from build123d import *

# Parameters (mm, degrees)
CBORE_FOR_M3_SHCS1_D           = 3.6
CBORE_FOR_M3_SHCS1_DEPTH       = 6.500114
CBORE_FOR_M3_SHCS1_CBORE_D     = 6.5
CBORE_FOR_M3_SHCS1_CBORE_DEPTH = 3
CBORE_FOR_M3_SHCS1_TIP         = 1.081549114
CUT_EXTRUDE1_DEPTH             = 91.160967098
CUT_EXTRUDE2_DEPTH             = 93.865494063


with BuildPart() as part:
    # Sketch1 → Revolve1 (revolve)
    with BuildSketch(Plane.XY, mode=Mode.PRIVATE) as revolve1_sk:
        Polygon((0, 83.999999926), (28, 83.999999926), (28, 78.999999926), (15, 78.999999926), (15, 79.999999926), (4.5, 79.999999926), (4.5, 15), (2.5, 15), (2.5, 0), (0, 0), align=None)
    revolve(revolve1_sk.sketch.rotate(Axis((0, 0, 0), (0, 1, 0)), 90), axis=Axis((0, 0, 0), (0, 1, 0)))

    # CBORE for M3 SHCS1
    with Locations(Plane(origin=(0, 83.999999926, 0), x_dir=(1, 0, 0), z_dir=(0, 1, 0))):
        with Locations((3, 23), (-3, 23), (-3, -23), (3, -23)):
            CounterBoreHole(CBORE_FOR_M3_SHCS1_D / 2, CBORE_FOR_M3_SHCS1_CBORE_D / 2, CBORE_FOR_M3_SHCS1_CBORE_DEPTH, depth=CBORE_FOR_M3_SHCS1_DEPTH)
            with Locations((0, 0, -(CBORE_FOR_M3_SHCS1_DEPTH + CBORE_FOR_M3_SHCS1_TIP / 2))):  # 118° drill point
                Cone(0, CBORE_FOR_M3_SHCS1_D / 2, CBORE_FOR_M3_SHCS1_TIP, mode=Mode.SUBTRACT)

    # Sketch4 → Cut-Extrude1 (cut, through all)
    with BuildSketch(Plane(origin=(0, 80.999999926, 0), x_dir=(1, 0, 0), z_dir=(0, 1, 0))):
        with BuildLine():
            Line((-3, 26.25), (3, 26.25))
            ThreePointArc((3, 26.25), (6.25, 23), (3, 19.75))
            Line((3, 19.75), (-3, 19.75))
            ThreePointArc((-3, 19.75), (-6.25, 23), (-3, 26.25))
        make_face()
        with BuildLine():
            Line((-3, -19.75), (3, -19.75))
            ThreePointArc((3, -19.75), (6.25, -23), (3, -26.25))
            Line((3, -26.25), (-3, -26.25))
            ThreePointArc((-3, -26.25), (-6.25, -23), (-3, -19.75))
        make_face()
    extrude(amount=CUT_EXTRUDE1_DEPTH, mode=Mode.SUBTRACT)

    # Sketch5 → Cut-Extrude2 (cut, through all)
    with BuildSketch(Plane(origin=(0, 83.999999926, 0), x_dir=(1, 0, 0), z_dir=(0, 1, 0))):
        with BuildLine():
            Line((-23.75, -9.5), (-23.75, 9.5))
            ThreePointArc((-23.75, 9.5), (-22.75, 10.5), (-21.75, 9.5))
            Line((-21.75, 9.5), (-21.75, -9.5))
            ThreePointArc((-21.75, -9.5), (-22.75, -10.5), (-23.75, -9.5))
        make_face()
    cut_extrude2 = extrude(amount=-CUT_EXTRUDE2_DEPTH, mode=Mode.SUBTRACT)

    # Mirror1: Cut-Extrude2 across plane
    add(cut_extrude2.mirror(Plane(origin=(0, 0, 0), x_dir=(0, 0, 1), z_dir=(1, 0, 0))), mode=Mode.SUBTRACT)


solid = part.part
Here's how the part is built. I have some questions about the finished solid (model axes, mm). A direction names the side the tool comes from. Coordinates: 2 decimals unless noted, no trailing zeros. Write each loop counter-clockwise with the first axis right and the second up, starting at its lowest first coordinate (ties: lowest second). Pieces come first, ordered by that corner, then holes.
1) Thinking about a two-plate mould opening in X: for faces 1 (the face through (2, 15, -2)), 2 (the face through (-0.1, 7.4, 2.5)), 3 (the face through (-22.7, 81.5, 10.5)), 4 (the face through (-6.25, 82.52, 22.93)), which applies, +X half, -X half, draft (parallel to the pull), parting line (faces both ways), or undercut?
Filled in:
face 1: draft
face 2: parting line
face 3: undercut
face 4: undercut
2) I'm going to push flat-ended pins straight in: pin 1 (5.5 mm diameter, centred on y = 82, z = 4, fed in from -X); pin 2 (4.5 mm diameter, centred on x = -3, z = 23, fed in from +Y); pin 3 (4 mm diameter, centred on y = 82, z = -4.5, fed in from +X). Where does each tip first touch, or does it pass through?
Filled in:
pin 1: stops at x = -27.97
pin 2: stops at y = 81
pin 3: stops at x = 27.89
3) If we section it at C-C (x = 22.75): List the corners of the cut face in (y, z) for me, plus the area to 3 significant figures.
Filled in:
outline: (79, -16.32) - (84, -16.32) - (84, -10.5) - (79, -10.5) - close; (79, 10.5) - (84, 10.5) - (84, 16.32) - (79, 16.32) - close
area: 58.2 mm2
4) If we section it at A-A (z = 0): List the corners of the cut face in (x, y) for me.
Filled in:
outline: (-28, 79) - (-23.75, 79) - (-23.75, 84) - (-28, 84) - close; (-21.75, 79) - (-15, 79) - (-15, 80) - (-4.5, 80) - (-4.5, 15) - (-2.5, 15) - (-2.5, 0) - (2.5, 0) - (2.5, 15) - (4.5, 15) - (4.5, 80) - (15, 80) - (15, 79) - (21.75, 79) - (21.75, 84) - (-21.75, 84) - close; (23.75, 79) - (28, 79) - (28, 84) - (23.75, 84) - close
5) If we section it at B-B (x = 0): List the corners of the cut face in (y, z) for me, plus the area to 3 significant figures.
Filled in:
outline: (0, -2.5) - (15, -2.5) - (15, -4.5) - (80, -4.5) - (80, -15) - (79, -15) - (79, -28) - (84, -28) - (84, -26.25) - (81, -26.25) - (81, -19.75) - (84, -19.75) - (84, 19.75) - (81, 19.75) - (81, 26.25) - (84, 26.25) - (84, 28) - (79, 28) - (79, 15) - (80, 15) - (80, 4.5) - (15, 4.5) - (15, 2.5) - (0, 2.5) - close
area: 871 mm2
6) Which directions (+Z, -Z, +X, -X, +Y, -Y) give clear straight access to the entire face, cutting with the end or side of a thin tool? Please do faces 5 (the face through (-23.75, 82, 0)), 6 (the face through (-12.65, 79.51, -8.06)), 7 (the face through (0, 82, -26.25)), 8 (the face through (0, 0, 0)).
Filled in:
face 5: +Y, -Y
face 6: -Y
face 7: +Y
face 8: +Z, -Z, +X, -X, -Y
7) If I drill on line 1 (X direction, y = 80, z = 23); line 2 (Y direction, x = 8, z = 19.5); line 3 (Y direction, x = -9, z = 1.5), over which ranges is the centre line in solid material (lowest first)?
Filled in:
line 1: x = -15.97 to -4.8, -1.2 to 1.2, 4.8 to 15.97
line 2: y = 79 to 84
line 3: y = 80 to 84
8) If we section it at D-D (y = 60.5): List the corners of the cut face in (x, z) for me.
Filled in:
outline: circle Ø9 at (0, 0)
